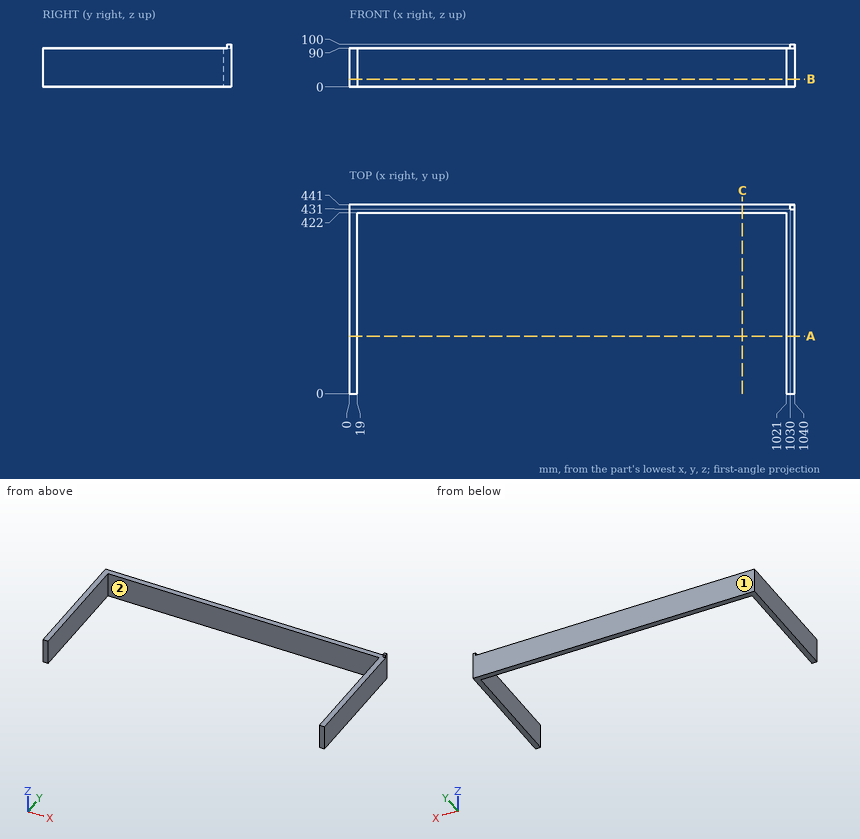
Can you work these out from the drawing? Everything is in mm from the part's minimum corner. Give positions to 0.01 mm unless a question says otherwise; leave off trailing zeros. Loops run counter-clockwise (first coordinate to the right, second up) from the corner with the lowest first, then second, coordinate; pieces in that order, holes last. Notation, with made-up numbers: (49, -24) -> (57, -24) arc R24 cw to (57, 0) -> close; hole circle Ø1 at (73, -1). An arc over 180 degrees is marked (long way). Return JSON: item names as keys, results as strings.
Q1. I want a section at B-B, the plane z = 18. List the corners of the cut face in (x, y) for me.
Checks:
{"outline": "(0, 0) -> (19, 0) -> (19, 422) -> (1021, 422) -> (1021, 0) -> (1040, 0) -> (1040, 441) -> (0, 441) -> close"}
Q2. I want a section at A-A, the plane y = 134. List the corners of the cut face in (x, z) for me, then the cut area to 3 significant figures.
Checks:
{"outline": "(0, 0) -> (19, 0) -> (19, 90) -> (0, 90) -> close; (1021, 0) -> (1040, 0) -> (1040, 90) -> (1021, 90) -> close", "area": "3,420 mm2"}
Q3. We'd pull the mould along X, two halves only. Please class the marked faces 1 and 2: released by +X, released by -X, zero draft, split by the parting line, or undercut.
Checks:
{"face 1": "zero draft", "face 2": "undercut"}
Q4. I want a section at C-C, the plane x = 918.5. List the corners of the cut face in (y, z) for me.
Checks:
{"outline": "(422, 0) -> (441, 0) -> (441, 90) -> (422, 90) -> close"}
Q5. For pin 1 Ø5 at (x, z) = (118.5, 64) entering from -Y; pin 2 Ø5 at (y, z) = (434, 94) entering from -X, each with a flat end and sliding along its axis, tell me the tip position at first contact or that it passes through.
Checks:
{"pin 1": "stops at y = 422", "pin 2": "stops at x = 1030"}
Q6. I need wall thicknesses on probe 1 along X at (y, z) = (96.5, 84.5); probe 2 along Y at (x, z) = (634, 75). Which ranges of each line are inside material? Lowest first, please.
Checks:
{"probe 1": "x = 0 to 19, 1021 to 1040", "probe 2": "y = 422 to 441"}
